```python
from build123d import *

# Parameters (mm, degrees)
SKETCH_1_R      = 1.65
EXTRUDE_1_DEPTH = 3
CHAMFER_1_SIZE  = 0.3


with BuildPart() as part:
    # 草图1 → 凸台-拉伸1 (new body)
    with BuildSketch(Plane.XY):
        with BuildLine():
            Line((-12.5, 3), (12.5, 3))
            ThreePointArc((12.5, 3), (15.5, 0), (12.5, -3))
            Line((12.5, -3), (-12.5, -3))
            ThreePointArc((-12.5, -3), (-15.5, 0), (-12.5, 3))
        make_face()
        with Locations((-12.5, 0)):
            Circle(SKETCH_1_R, mode=Mode.SUBTRACT)
        with Locations((12.5, 0)):
            Circle(SKETCH_1_R, mode=Mode.SUBTRACT)
    extrude(amount=EXTRUDE_1_DEPTH)

    # 倒角1
    chamfer_1_edges = [part.edges().sort_by_distance(p)[0] for p in [
        (-14.15, 0, 0),
        (15.5, 0, 3),
        (10.85, 0, 0),
        (0, 3, 3),
        (-15.5, 0, 3),
        (0, 3, 0),
        (15.5, 0, 0),
        (0, -3, 0),
        (-15.5, 0, 0),
        (0, -3, 3),
    ]]
    chamfer(chamfer_1_edges, length=CHAMFER_1_SIZE)


solid = part.part
```
Design review of the part built by this model. Coordinates are the model's own, in mm. Coordinates: 2 decimals unless noted, no trailing zeros. Write each loop counter-clockwise with the first axis right and the second up, starting at its lowest first coordinate (ties: lowest second). Pieces come first, ordered by that corner, then holes. Notation, with made-up numbers: M 67.5,-16 L 111.5,-16 A25 ccw 111.5,9 Z; hole C 44,64 d6. An arc over 180 degrees is marked long. Answer as a JSON object with one key per item and string values.
Item 1: Add section C-C, the plane y = -1.2. State how many separate pieces and enclosed holes the cut face has, and give its area (3 significant figures).
Outcome:
{"separate pieces": "3", "enclosed holes": "0", "area": "77.5 mm²"}
Item 2: Wall thickness on probe 1 along X at (y, z) = (-0.1, 1.1); probe 2 along X at (y, z) = (-1.2, 0.95); probe 3 along Y at (x, z) = (-12.5, 2.05): over which ranges is each line inside the solid? List them lowest first.
Outcome:
{"probe 1": "-15.5 to -14.15, -10.85 to 10.85, 14.15 to 15.5", "probe 2": "-15.25 to -13.63, -11.37 to 11.37, 13.63 to 15.25", "probe 3": "-3 to -1.65, 1.65 to 3"}
Item 3: Insertion check: pin 1 Ø1.5 at (y, z) = (0.5, 2.5) entering from +X. The pin has a flat end and moves straight along its axis. Give the tip position at first contact, or say it passes through.
Outcome:
{"pin 1": "x = 15.5"}
Item 4: Draft analysis for pull direction Y (two halves, no side actions). For faces 1 (the flat face through (0, 3, 1)), 2 (the conical face through (-15.31, -0.06, 0.11)), 3 (the cylindrical face through (14.024, -0.632, 1.631)), 4 (the cylindrical face through (-10.976, -0.632, 1.631)), state which applies: pulls with the +Y half, pulls with the -Y half, needs draft (parallel to the pull), parting line crosses it, or undercut.
Outcome:
{"face 1": "pulls with the +Y half", "face 2": "parting line crosses it", "face 3": "undercut", "face 4": "undercut"}
Item 5: Add section A-A, the plane y = 0. Give the boundary of the cut face in (x, z).
Outcome:
{"outline": "M -15.5,0.3 L -15.2,0 L -14.45,0 L -14.15,0.3 L -14.15,3 L -15.2,3 L -15.5,2.7 Z; M -10.85,0.3 L -10.55,0 L 10.55,0 L 10.85,0.3 L 10.85,3 L -10.85,3 Z; M 14.15,0.3 L 14.45,0 L 15.2,0 L 15.5,0.3 L 15.5,2.7 L 15.2,3 L 14.15,3 Z"}
Item 6: Add section B-B, the plane z = 2.15. Give the boundary of the cut face in (x, y), and give its area (3 significant figures).
Outcome:
{"outline": "M -12.5,-3 L 12.5,-3 A3 ccw 12.5,3 L -12.5,3 A3 ccw Z; hole C -12.5,0 d3.3; hole C 12.5,0 d3.3", "area": "161 mm²"}
